Could you check a few things on this model? Use its own coordinates, in mm. Face numbers are marked on the shaded views. A direction names the side the tool comes from. Coordinates: 2 decimals unless noted, no trailing zeros. Loops run counter-clockwise (first coordinate to the right, second up) from the corner with the lowest first, then second, coordinate; pieces in that order, holes last.
Autodesk Inventor part; units mm, degrees
ref_plane "YZ Plane" through (0, 0, 0) normal (1, 0, 0) x (0, 1, 0)
ref_plane "XZ Plane" through (0, 0, 0) normal (0, 1, 0) x (-1, 0, 0)
ref_plane "XY Plane" through (0, 0, 0) normal (0, 0, 1) x (1, 0, 0)
sketch "Sketch1" plane through (0, 0, 0) normal (0, 0, 1) x (1, 0, 0)
  line L0 (-11, -30) -> (11, -30)
  line L1 (11, -30) -> (11, 30)
  line L2 (11, 30) -> (-11, 30)
  line L3 (-11, 30) -> (-11, -30)
  circle A0 centre (-8, 0) radius 2.25
  line L4 (-5, 30) -> (-5, -30) construction
  line L5 (5, 30) -> (5, -30) construction
  line L6 (0, 30) -> (0, -30) construction
  circle A1 centre (-8, 27) radius 2.25
  circle A2 centre (-8, -27) radius 2.25
  circle A3 centre (8, -27) radius 2.25
  circle A4 centre (8, 0) radius 2.25
  circle A5 centre (8, 27) radius 2.25
  line L7 (-11, 0) -> (11, 0) construction
  line L8 (-11, 30) -> (11, 30)
  line L9 (11, 30) -> (11, 24)
  line L10 (11, 24) -> (-11, 24)
  line L11 (-11, 24) -> (-11, 30)
  line L12 (-11, 3) -> (11, 3)
  line L13 (11, 3) -> (11, -3)
  line L14 (11, -3) -> (-11, -3)
  line L15 (-11, -3) -> (-11, 3)
  line L16 (-11, -30) -> (11, -30)
  line L17 (11, -30) -> (11, -24)
  line L18 (11, -24) -> (-11, -24)
  line L19 (-11, -24) -> (-11, -30)
  point P0 (0, 0)
  dimension "d0" = 4.5
  dimension "d1" = 3
  dimension "d2" = 3
  dimension "d3" = 10
  dimension "d4" = 60
  dimension "d5" = 4.5
  dimension "d6" = 3
  dimension "d7" = 3
  dimension "d8" = 4.5
  dimension "d9" = 3
  dimension "d10" = 3
  dimension "d11" = 3
  dimension "d14" = 58.5
  dimension "d15" = 3
  dimension "d16" = 3
  dimension "d17" = 3
  dimension "d18" = 3
extrude "Extrusion1" add sketch "Sketch1" along normal blind 0.6
extrude "Extrusion2" add sketch "Sketch1" along normal blind 1.2 contours L3 L18 L1 L0 | L3 L12 L1 L14 | L3 L2 L1 L10
properties part number "FoldLink"
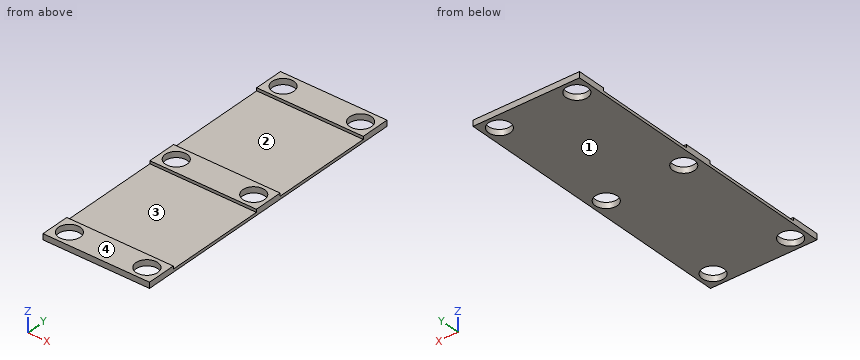
(1) Imagine slicing it at C-C, the plane z = 0.25. Write out the boundary of the cut face in (x, y).
Answers:
outline: (-11, -30) - (11, -30) - (11, 30) - (-11, 30) - close; hole circle Ø4.5 at (-8, -27); hole circle Ø4.5 at (-8, 0); hole circle Ø4.5 at (-8, 27); hole circle Ø4.5 at (8, -27); hole circle Ø4.5 at (8, 0); hole circle Ø4.5 at (8, 27)
(2) For pin 1 (6.5 mm diameter, centred on x = -1, y = -14, fed in from +Z), with a flat end and sliding along its axis, tell me the tip position at first contact or that it passes through.
Answers:
pin 1: stops at z = 0.6
(3) Which directions (+Z, -Z, +X, -X, +Y, -Y) give clear straight access to the entire face, cutting with the end or side of a thin tool? Please do the marked faces 1 and 2.
Answers:
face 1: -Z, +X, -X, +Y, -Y
face 2: +Z, +X, -X
(4) We'd pull the mould along Y, two halves only. Please class the marked faces 3 and 4: +Y half, -Y half, draft (parallel to the pull), parting line (faces both ways), or undercut.
Answers:
face 3: undercut
face 4: draft
(5) Imagine slicing it at B-B, the plane y = -27. Write out the boundary of the cut face in (x, z), and give its area (3 significant figures).
Answers:
outline: (-11, 0) - (-10.25, 0) - (-10.25, 1.2) - (-11, 1.2) - close; (-5.75, 0) - (5.75, 0) - (5.75, 1.2) - (-5.75, 1.2) - close; (10.25, 0) - (11, 0) - (11, 1.2) - (10.25, 1.2) - close
area: 15.6 mm2
(6) I need wall thicknesses on probe 1 along Y at (x, z) = (-8, 0.4); probe 2 along Y at (x, z) = (-8, 1); probe 3 along Y at (x, z) = (9.5, 0.4). Which ranges of each line are inside material? Lowest first, please.
Answers:
probe 1: y = -30 to -29.25, -24.75 to -2.25, 2.25 to 24.75, 29.25 to 30
probe 2: y = -30 to -29.25, -24.75 to -24, -3 to -2.25, 2.25 to 3, 24 to 24.75, 29.25 to 30
probe 3: y = -30 to -28.68, -25.32 to -1.68, 1.68 to 25.32, 28.68 to 30
(7) Imagine slicing it at A-A, the plane x = 8. Write out the boundary of the cut face in (y, z).
Answers:
outline: (-30, 0) - (-29.25, 0) - (-29.25, 1.2) - (-30, 1.2) - close; (-24.75, 0) - (-2.25, 0) - (-2.25, 1.2) - (-3, 1.2) - (-3, 0.6) - (-24, 0.6) - (-24, 1.2) - (-24.75, 1.2) - close; (2.25, 0) - (24.75, 0) - (24.75, 1.2) - (24, 1.2) - (24, 0.6) - (3, 0.6) - (3, 1.2) - (2.25, 1.2) - close; (29.25, 0) - (30, 0) - (30, 1.2) - (29.25, 1.2) - close
(8) Imagine slicing it at D-D, the plane x = -1.75. Write out the boundary of the cut face in (y, z), and give its area (3 significant figures).
Answers:
outline: (-30, 0) - (30, 0) - (30, 1.2) - (24, 1.2) - (24, 0.6) - (3, 0.6) - (3, 1.2) - (-3, 1.2) - (-3, 0.6) - (-24, 0.6) - (-24, 1.2) - (-30, 1.2) - close
area: 46.8 mm2
